Check sheet for the drawn part. Datum: minimum x, y, z corner. Units: mm. Round coordinates to 2 decimals unless told otherwise and drop trailing zeros. Order: outer loops, then holes, each group sorted by start corner. A loop starts at its lowest first (then second) coordinate and runs counter-clockwise, first axis right, second up. Notation, with made-up numbers: M 65.25,-34 L 123.25,-34 A16 ccw 123.25,-12 Z; hole C 88,42 d11. An arc over 180 degrees is marked long. Use one line per item in the form item = value. Start each with the question number.
Item 1: Cross-section at B-B on y = 91. Enter the section's corners in (x, z), then the cut area to 3 significant figures.
Item 2: Cross-section at D-D on y = 165.1. Enter the section's corners in (x, z), then the cut area to 3 significant figures.
Item 3: Cross-section at A-A on x = 88.9. Enter the section's corners in (y, z), then the cut area to 3 significant figures.
Item 4: Cross-section at C-C on z = 7.25. Enter the section's corners in (x, y).
Item 5: Release check for a two-part mould opening along Y. For the marked faces 1 and 2 record: +Y half, -Y half, draft (parallel to the pull), parting line (faces both ways), or undercut.
Item 6: Thickness scan on probe 1 along Y at (x, z) = (88.9, 1.45); probe 2 along Z at (x, y) = (127.5, 101); probe 3 along X at (y, z) = (130.5, 0.75). Record the ranges inside material, lowest first. Write a range as [from, to].
Item 7: Go/stop test with a flat-tipped pin: pin 1 Ø1.5 at (x, y) = (34, 32.5) entering from +Z. Record where the tip stops, or that it passes through.
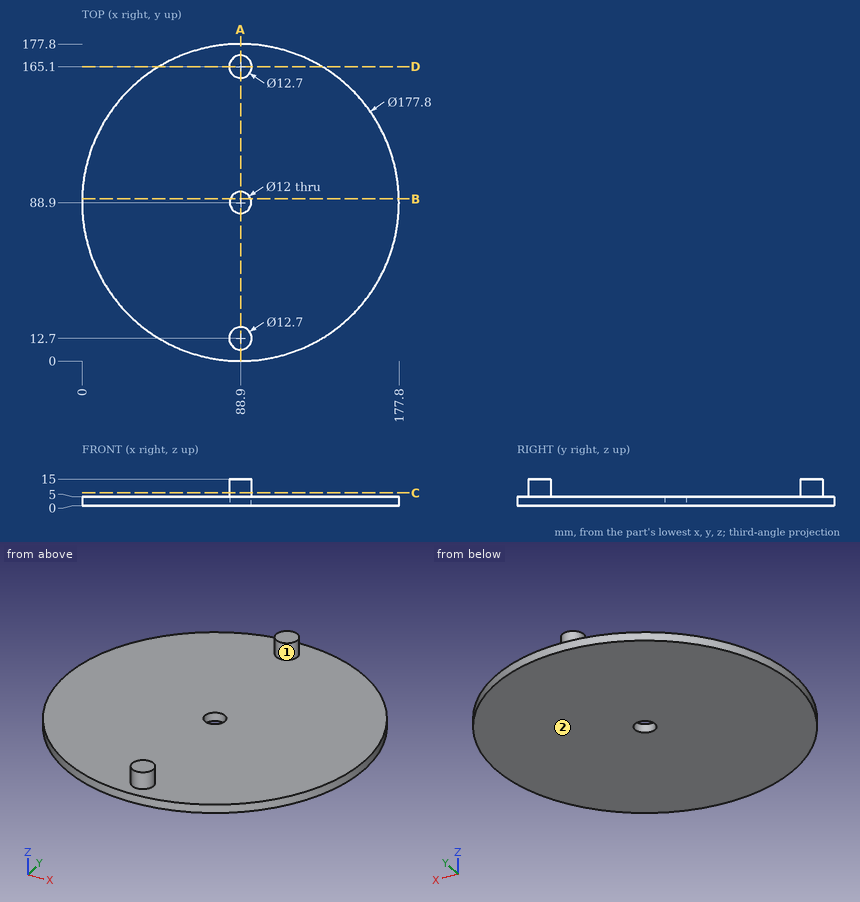
Output values:
q1.outline = M 0.02,0 L 83.28,0 L 83.28,5 L 0.02,5 Z; M 94.52,0 L 177.78,0 L 177.78,5 L 94.52,5 Z
q1.area = 833 mm2
q2.outline = M 43.11,0 L 134.69,0 L 134.69,5 L 95.25,5 L 95.25,15 L 82.55,15 L 82.55,5 L 43.11,5 Z
q2.area = 585 mm2
q3.outline = M 0,0 L 82.9,0 L 82.9,5 L 19.05,5 L 19.05,15 L 6.35,15 L 6.35,5 L 0,5 Z; M 94.9,0 L 177.8,0 L 177.8,5 L 171.45,5 L 171.45,15 L 158.75,15 L 158.75,5 L 94.9,5 Z
q3.area = 1,080 mm2
q4.outline = C 88.9,12.7 d12.7; C 88.9,165.1 d12.7
q5.face_1 = undercut
q5.face_2 = draft
q6.probe_1 = [0, 82.9], [94.9, 177.8]
q6.probe_2 = [0, 5]
q6.probe_3 = [10.33, 167.47]
q7.pin_1 = 5
